CAD build for the part. Positions are in the model's coordinates, mm. Round coordinates to 2 decimals unless told otherwise and drop trailing zeros. Order: outer loops, then holes, each group sorted by start corner. A loop starts at its lowest first (then second) coordinate and runs counter-clockwise, first axis right, second up. Notation, with made-up numbers: M -23,21 L 30,21 A22 cw 30,37 Z; hole C 49,-17 d4. An arc over 180 degrees is marked long. Answer as a JSON object with one key per item and string values. Group by question number.
```python
from build123d import *

# Parameters (mm, degrees)
SKETCH1_W               = 482.6
SKETCH1_H               = 330.2
BOSS_EXTRUDE1_DEPTH     = 12.7
CUT_EXTRUDE1_DEPTH      = 293.651652994
CUT_EXTRUDE1_DEPTH_BACK = 293.651652994
SKETCH2_R               = 4.7625
CUT_EXTRUDE2_DEPTH      = 293.651652994
CUT_EXTRUDE2_DEPTH_BACK = 293.651652994
SKETCH4_R               = 8.636


with BuildPart() as part:
    # Sketch1 → Boss-Extrude1 (new body)
    with BuildSketch(Plane(origin=(0, 0, 0), x_dir=(1, 0, 0), z_dir=(0, 1, 0))):
        Rectangle(SKETCH1_W, SKETCH1_H)
    extrude(amount=BOSS_EXTRUDE1_DEPTH)

    # Sketch2 → Cut-Extrude1 (cut, two sides: drawn at the far end of the back side and taken through both)
    with BuildSketch(Plane(origin=(0, 12.7, 0), x_dir=(1, 0, 0), z_dir=(0, 1, 0)).offset(-CUT_EXTRUDE1_DEPTH_BACK)):
        with Locations(Location((215.9, 146.05, 0), (0, 0, 270))):
            Circle(SKETCH2_R)
        with Locations(Location((-215.9, 146.05, 0), (0, 0, 270))):
            Circle(SKETCH2_R)
        with Locations(Location((215.9, -146.05, 0), (0, 0, 270))):
            Circle(SKETCH2_R)
        with Locations(Location((-215.9, -146.05, 0), (0, 0, 270))):
            Circle(SKETCH2_R)
        with Locations(Location((0, 146.05, 0), (0, 0, 270))):
            Circle(SKETCH2_R)
        with Locations(Location((0, -146.05, 0), (0, 0, 270))):
            Circle(SKETCH2_R)
    extrude(amount=CUT_EXTRUDE1_DEPTH + CUT_EXTRUDE1_DEPTH_BACK, mode=Mode.SUBTRACT)

    # Sketch4 → Cut-Extrude2 (cut, two sides: drawn at the far end of the back side and taken through both)
    with BuildSketch(Plane(origin=(0, 12.7, 0), x_dir=(1, 0, 0), z_dir=(0, 1, 0)).offset(-CUT_EXTRUDE2_DEPTH_BACK)):
        with Locations(Location((-25.4, 76.2, 0), (0, 0, 270))):
            Circle(SKETCH4_R)
        with Locations(Location((25.4, 76.2, 0), (0, 0, 270))):
            Circle(SKETCH4_R)
        with Locations(Location((76.2, 76.2, 0), (0, 0, 270))):
            Circle(SKETCH4_R)
        with Locations(Location((127, 76.2, 0), (0, 0, 270))):
            Circle(SKETCH4_R)
        with Locations(Location((127, -76.2, 0), (0, 0, 270))):
            Circle(SKETCH4_R)
        with Locations(Location((76.2, -76.2, 0), (0, 0, 270))):
            Circle(SKETCH4_R)
        with Locations(Location((25.4, -76.2, 0), (0, 0, 270))):
            Circle(SKETCH4_R)
        with Locations(Location((-25.4, -76.2, 0), (0, 0, 270))):
            Circle(SKETCH4_R)
    extrude(amount=CUT_EXTRUDE2_DEPTH + CUT_EXTRUDE2_DEPTH_BACK, mode=Mode.SUBTRACT)


solid = part.part
```
Item 1: Two-plate mould, pull along X, no slides. Class faces 1 (the face through (216.109, 6.261, -150.808)), 2 (the face through (-3, 0, -2)), 3 (the face through (-241.3, 6, 2)): +X half, -X half, draft (parallel to the pull), parting line (faces both ways), or undercut.
Item 2: Flat gauge pin, fed straight in: pin 1 Ø10.5 at (x, z) = (127, 76.2) entering from +Y. Where does the tip first touch, or does it go through?
Item 3: Cut at B-B, the plane x = 215.9. Give the cut face in (y, z).
Item 4: Cut at A-A, the plane z = -146.05. Give the cut face in (x, y).
Item 5: Drill centre lines: line 1 (X direction, y = 6.5, z = -76.2); line 2 (Z direction, x = 215.9, y = 7.5); line 3 (X direction, y = 2.5, z = -146.05). Where is each one in solid material? Low to high. Write a range as [from, to].
Item 6: Cut at C-C, the plane z = 76.2. Give the cut face in (x, y).
Item 7: Cut at D-D, the plane x = -25.4. Give the cut face in (y, z).
Response values:
{
 "1": {"face 1": "undercut", "face 2": "draft", "face 3": "-X half"},
 "2": {"pin 1": "through"},
 "3": {"outline": "M 0,-165.1 L 12.7,-165.1 L 12.7,-150.81 L 0,-150.81 Z; M 0,-141.29 L 12.7,-141.29 L 12.7,141.29 L 0,141.29 Z; M 0,150.81 L 12.7,150.81 L 12.7,165.1 L 0,165.1 Z"},
 "4": {"outline": "M -241.3,0 L -220.66,0 L -220.66,12.7 L -241.3,12.7 Z; M -211.14,0 L -4.76,0 L -4.76,12.7 L -211.14,12.7 Z; M 4.76,0 L 211.14,0 L 211.14,12.7 L 4.76,12.7 Z; M 220.66,0 L 241.3,0 L 241.3,12.7 L 220.66,12.7 Z"},
 "5": {"line 1": "[-241.3, -34.04], [-16.76, 16.76], [34.04, 67.56], [84.84, 118.36], [135.64, 241.3]", "line 2": "[-165.1, -150.81], [-141.29, 141.29], [150.81, 165.1]", "line 3": "[-241.3, -220.66], [-211.14, -4.76], [4.76, 211.14], [220.66, 241.3]"},
 "6": {"outline": "M -241.3,0 L -34.04,0 L -34.04,12.7 L -241.3,12.7 Z; M -16.76,0 L 16.76,0 L 16.76,12.7 L -16.76,12.7 Z; M 34.04,0 L 67.56,0 L 67.56,12.7 L 34.04,12.7 Z; M 84.84,0 L 118.36,0 L 118.36,12.7 L 84.84,12.7 Z; M 135.64,0 L 241.3,0 L 241.3,12.7 L 135.64,12.7 Z"},
 "7": {"outline": "M 0,-165.1 L 12.7,-165.1 L 12.7,-84.84 L 0,-84.84 Z; M 0,-67.56 L 12.7,-67.56 L 12.7,67.56 L 0,67.56 Z; M 0,84.84 L 12.7,84.84 L 12.7,165.1 L 0,165.1 Z"}
}
